The model under review builds one solid part; all positions refer to its coordinate system, in mm. Face numbers are marked on the shaded views. A direction names the side the tool comes from. Round coordinates to 2 decimals unless told otherwise and drop trailing zeros. Order: outer loops, then holes, each group sorted by start corner. A loop starts at its lowest first (then second) coordinate and runs counter-clockwise, first axis right, second up.
```python
from build123d import *

# Parameters (mm, degrees)
EXTRUDE1_DEPTH = 6.223
SKETCH2_R      = 4.699
EXTRUDE2_DEPTH = 88.9
CHAMFER1_SIZE  = 0.3962


with BuildPart() as part:
    # Sketch1 → Extrude1 (new body)
    with BuildSketch(Plane(origin=(0, 0, 0), x_dir=(1, 0, 0), z_dir=(0, 1, 0))):
        Polygon((8.263556668, 0), (4.131778334, 7.15645), (-4.131778334, 7.15645), (-8.263556668, 0), (-4.131778334, -7.15645), (4.131778334, -7.15645), align=None)
    extrude(amount=-EXTRUDE1_DEPTH)

    # Sketch2 → Extrude2 (add)
    with BuildSketch(Plane.XZ.offset(6.223)):
        with Locations(Location((0, 0, 0), (0, 0, 90))):
            Circle(SKETCH2_R)
    extrude(amount=EXTRUDE2_DEPTH)

    # Chamfer1
    chamfer1_edges = [part.edges().sort_by_distance(p)[0] for p in [
        (0, -95.123, -4.699),
    ]]
    chamfer(chamfer1_edges, length=CHAMFER1_SIZE)


solid = part.part
```
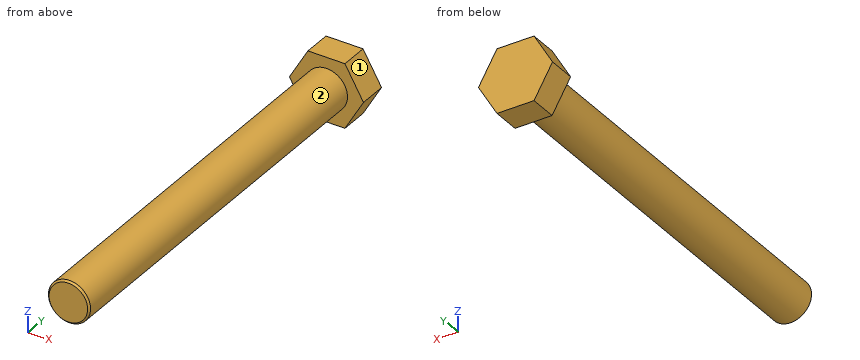
(1) Consider section C-C (z = -5.5). Write out the cut boundary in (x, y), and give its area (3 significant figures).
Data:
outline: (-5.09, -6.22) - (5.09, -6.22) - (5.09, 0) - (-5.09, 0) - close
area: 63.3 mm2
(2) Consider section B-B (y = -57.5). Write out the cut boundary in (x, z).
Data:
outline: circle Ø9.4 at (0, 0)
(3) For the marked faces 1 and 2, list the 3-axis set-ups (+Z, -Z, +X, -X, +Y, -Y) from which the entire face can be reached by the end or side of a thin tool; tool diameter is ignored.
Data:
face 1: +Z, +X, +Y, -Y
face 2: -Y
(4) Insertion check: pin 1 (6 mm diameter, centred on x = -3, y = -48, fed in from +Z); pin 2 (5 mm diameter, centred on x = 2.5, y = -35, fed in from -Z); pin 3 (7 mm diameter, centred on x = 4, z = 2.5, fed in from -Y); pin 4 (2 mm diameter, centred on x = -2.5, y = -64.5, fed in from -Z). Each pin has a flat end and moves straight along its axis. Give the tip position at first contact, or say it passes through.
Data:
pin 1: stops at z = 4.7
pin 2: stops at z = -4.7
pin 3: stops at y = -95.12
pin 4: stops at z = -4.45
(5) Consider section D-D (x = -6.25). Write out the cut boundary in (y, z).
Data:
outline: (-6.22, -3.49) - (0, -3.49) - (0, 3.49) - (-6.22, 3.49) - close
(6) To check wall thickness, follow probe 1 along Y at (x, z) = (6.75, 0.5); probe 2 along Z at (x, y) = (1, -62); probe 3 along Z at (x, y) = (3.75, -55.5). State the ranges of each line that lie inside material, in increasing order.
Data:
probe 1: y = -6.22 to 0
probe 2: z = -4.59 to 4.59
probe 3: z = -2.83 to 2.83
(7) Consider section A-A (x = 0). Write out the cut boundary in (y, z), and give its area (3 significant figures).
Data:
outline: (-95.12, -4.3) - (-94.73, -4.7) - (-6.22, -4.7) - (-6.22, -7.16) - (0, -7.16) - (0, 7.16) - (-6.22, 7.16) - (-6.22, 4.7) - (-94.73, 4.7) - (-95.12, 4.3) - close
area: 924 mm2
